Geometry: final body of the model. Coordinates: model frame, mm. Face numbers are marked on the shaded views. A direction names the side the tool comes from. Coordinates: 2 decimals unless noted, no trailing zeros. Order: outer loops, then holes, each group sorted by start corner. A loop starts at its lowest first (then second) coordinate and runs counter-clockwise, first axis right, second up. Notation, with made-up numbers: (83.5, 67) -> (97.5, 67) arc R9 ccw to (97.5, 81) -> close; hole circle Ø6 at (-37.75, 26.5). An arc over 180 degrees is marked (long way). Use one line per item in the form item = value.
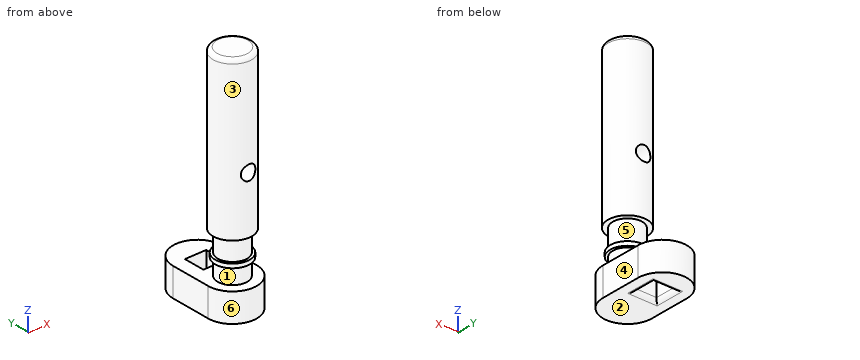
```python
from build123d import *

# Parameters (mm, degrees)
SKETCH1_W           = 5.288
SKETCH1_H           = 5.288
BOSS_EXTRUDE1_DEPTH = 7
FILLET1_R           = 1
FILLET2_R           = 1
SKETCH6_R           = 1.8
CUT_EXTRUDE1_DEPTH  = 58.661920682


with BuildPart() as part:
    # Sketch1 → Boss-Extrude1 (new body)
    with BuildSketch(Plane.XY):
        with BuildLine():
            Line((6, 0), (6, -10))
            ThreePointArc((6, -10), (0, -16), (-6, -10))
            Line((-6, -10), (-6, 0))
            ThreePointArc((-6, 0), (0, 6), (6, 0))
        make_face()
        with Locations((0, -2.1)):
            Rectangle(SKETCH1_W, SKETCH1_H, mode=Mode.SUBTRACT)
    extrude(amount=BOSS_EXTRUDE1_DEPTH)

    # Sketch4 → Revolve1 (revolve)
    with BuildSketch(Plane(origin=(0, 0, 0), x_dir=(0, 0, -1), z_dir=(1, 0, 0)), mode=Mode.PRIVATE) as revolve1_sk:
        Polygon((-7, -13.625), (-11, -13.625), (-11, -14.264510891), (-12, -14.264510891), (-12, -13.625), (-17.25, -13.625), (-17.25, -14.264510891), (-17.25, -14.8), (-20.259244151, -14.8), (-56.24461838, -14.8), (-56.24461838, -13.625), (-56.24461838, -10), (-7, -10), align=None)
    revolve(revolve1_sk.sketch.rotate(Axis((0, -10, 7), (0, 0, 1)), 180), axis=Axis((0, -10, 7), (0, 0, 1)))

    # Fillet1
    fillet1_edges = [part.edges().sort_by_distance(p)[0] for p in [
        (2.644, -2.1, 0),
        (0, 0.544, 0),
        (-2.644, -2.1, 0),
        (0, -4.744, 0),
    ]]
    fillet(fillet1_edges, radius=FILLET1_R)

    # Fillet2
    fillet2_edges = [part.edges().sort_by_distance(p)[0] for p in [
        (0, -14.8, 56.24461838),
    ]]
    fillet(fillet2_edges, radius=FILLET2_R)

    # Sketch6 → Cut-Extrude1 (cut, through all)
    with BuildSketch(Plane(origin=(0, -5.2, 0), x_dir=(1, 0, 0), z_dir=(0, 1, 0))):
        with Locations(Location((0, -31.24461838, 0), (0, 0, 270))):
            Circle(SKETCH6_R)
    extrude(amount=-CUT_EXTRUDE1_DEPTH, mode=Mode.SUBTRACT)


solid = part.part
```
1) Material intervals for probe 1 along Z at (x, y) = (-3, -7.5); probe 2 along Z at (x, y) = (0, -13.5); probe 3 along Z at (x, y) = (0.5, 3.25), sorted ascending. Write a range as from..to.
Results found:
probe_1 = 0..7, 11..12, 17.25..56.24
probe_2 = 0..29.44, 33.04..56.24
probe_3 = 0..7
2) Access query for the marked faces 1, 2 and 3. Directions: +Z, -Z, +X, -X, +Y, -Y. A direction counts if a zero-diameter tool reaches every point of the face in a straight line with its end or side. Return the directions, or none.
Results found:
face_1 = none
face_2 = -Z, +X, -X, +Y, -Y
face_3 = +Z
3) Section B-B, the plane z = 4.5. Output: boundary loops of the cut face in (x, y).
Results found:
outline = (-6, -10) arc R6 ccw to (6, -10) -> (6, 0) arc R6 ccw to (-6, 0) -> close; hole (-2.64, -4.74) -> (2.64, -4.74) -> (2.64, 0.54) -> (-2.64, 0.54) -> close
4) Section C-C, the plane z = 51.5. Output: boundary loops of the cut face in (x, y).
Results found:
outline = circle Ø9.6 at (0, -10)
5) Contact query for flat-ended pins moving along their axis: P1, Ø6, axis at y = -6.5, z = 14, coming from the +X side; P2, Ø12, axis at y = -4, z = 42.5, coming from the -X side; P3, Ø1.6, axis at x = 1, z = 4, coming from the -Y side. Output: stop coordinate, or through.
Results found:
P1 = 4.07
P2 = -4.8
P3 = -16
6) Pull-direction query (Y, two-part tool) for the marked faces 4, 5 and 6; classes: released by +Y, released by -Y, zero draft, split by the parting line, or undercut.
Results found:
face_4 = zero draft
face_5 = split by the parting line
face_6 = released by -Y
7) Section A-A, the plane x = 0. Give the number of separate pieces and of enclosed holes in the cut face, and give its area (3 significant figures).
Results found:
separate_pieces = 3
enclosed_holes = 0
area = 532 mm2
